```python
from build123d import *

# Parameters (mm, degrees)
SKETCH1_R           = 2.1
BOSS_EXTRUDE1_DEPTH = 500


with BuildPart() as part:
    # Sketch1 → Boss-Extrude1 (new body)
    with BuildSketch(Plane(origin=(0, 0, 0), x_dir=(-1, 0, 0), z_dir=(0, 0, -1))):
        with BuildLine():
            Line((-9.646446609, -22.821446609), (-7.771446609, -20.946446609))
            ThreePointArc((-7.771446609, -20.946446609), (-7.663060234, -20.784234935), (-7.625, -20.592893219))
            Line((-7.625, -20.592893219), (-7.625, -20.5))
            ThreePointArc((-7.625, -20.5), (-7.478553391, -20.146446609), (-7.125, -20))
            Line((-7.125, -20), (-3.3, -20))
            ThreePointArc((-3.3, -20), (-3.087867966, -19.912132034), (-3, -19.7))
            Line((-3, -19.7), (-3, -18))
            Line((-3, -18), (-6, -18))
            Line((-6, -18), (-6, -17.060660172))
            Line((-6, -17.060660172), (-2.939339828, -14))
            Line((-2.939339828, -14), (-0.3, -14))
            Line((-0.3, -14), (0, -13.7))
            Line((0, -13.7), (0.3, -14))
            Line((0.3, -14), (2.939339828, -14))
            Line((2.939339828, -14), (6, -17.060660172))
            Line((6, -17.060660172), (6, -18))
            Line((6, -18), (3, -18))
            Line((3, -18), (3, -19.7))
            ThreePointArc((3, -19.7), (3.087867966, -19.912132034), (3.3, -20))
            Line((3.3, -20), (9, -20))
            ThreePointArc((9, -20), (9.707106781, -19.707106781), (10, -19))
            Line((10, -19), (10, -13.3))
            ThreePointArc((10, -13.3), (9.912132034, -13.087867966), (9.7, -13))
            Line((9.7, -13), (8, -13))
            Line((8, -13), (8, -16))
            Line((8, -16), (7.060660172, -16))
            Line((7.060660172, -16), (4, -12.939339828))
            Line((4, -12.939339828), (4, -10.3))
            Line((4, -10.3), (3.7, -10))
            Line((3.7, -10), (4, -9.7))
            Line((4, -9.7), (4, -7.060660172))
            Line((4, -7.060660172), (7.060660172, -4))
            Line((7.060660172, -4), (8, -4))
            Line((8, -4), (8, -7))
            Line((8, -7), (9.7, -7))
            ThreePointArc((9.7, -7), (9.912132034, -6.912132034), (10, -6.7))
            Line((10, -6.7), (10, 6.7))
            ThreePointArc((10, 6.7), (9.912132034, 6.912132034), (9.7, 7))
            Line((9.7, 7), (8, 7))
            Line((8, 7), (8, 4))
            Line((8, 4), (7.060660172, 4))
            Line((7.060660172, 4), (4, 7.060660172))
            Line((4, 7.060660172), (4, 9.7))
            Line((4, 9.7), (3.7, 10))
            Line((3.7, 10), (4, 10.3))
            Line((4, 10.3), (4, 12.939339828))
            Line((4, 12.939339828), (7.060660172, 16))
            Line((7.060660172, 16), (8, 16))
            Line((8, 16), (8, 13))
            Line((8, 13), (9.7, 13))
            ThreePointArc((9.7, 13), (9.912132034, 13.087867966), (10, 13.3))
            Line((10, 13.3), (10, 19))
            ThreePointArc((10, 19), (9.707106781, 19.707106781), (9, 20))
            Line((9, 20), (3.300000001, 20))
            ThreePointArc((3.300000001, 20), (3.087867966, 19.912132034), (3, 19.699999999))
            Line((3, 19.699999999), (3, 18))
            Line((3, 18), (6, 18))
            Line((6, 18), (6, 17.060660172))
            Line((6, 17.060660172), (2.939339828, 14))
            Line((2.939339828, 14), (0.3, 14))
            Line((0.3, 14), (0, 13.7))
            Line((0, 13.7), (-0.3, 14))
            Line((-0.3, 14), (-2.939339828, 14))
            Line((-2.939339828, 14), (-6, 17.060660172))
            Line((-6, 17.060660172), (-6, 18))
            Line((-6, 18), (-3, 18))
            Line((-3, 18), (-3, 19.7))
            ThreePointArc((-3, 19.7), (-3.087867966, 19.912132034), (-3.3, 20))
            Line((-3.3, 20), (-7.125, 20))
            ThreePointArc((-7.125, 20), (-7.478553391, 20.146446609), (-7.625, 20.5))
            Line((-7.625, 20.5), (-7.625, 20.592893219))
            ThreePointArc((-7.625, 20.592893219), (-7.663060234, 20.784234935), (-7.771446609, 20.946446609))
            Line((-7.771446609, 20.946446609), (-9.646446609, 22.821446609))
            ThreePointArc((-9.646446609, 22.821446609), (-10, 22.967893219), (-10.353553391, 22.821446609))
            Line((-10.353553391, 22.821446609), (-12.228553391, 20.946446609))
            ThreePointArc((-12.228553391, 20.946446609), (-12.336939766, 20.784234935), (-12.375, 20.592893219))
            Line((-12.375, 20.592893219), (-12.375, 20))
            Line((-12.375, 20), (-10, 20))
            Line((-10, 20), (-10, 13.3))
            ThreePointArc((-10, 13.3), (-9.912132034, 13.087867966), (-9.7, 13))
            Line((-9.7, 13), (-8, 13))
            Line((-8, 13), (-8, 16))
            Line((-8, 16), (-7.060660172, 16))
            Line((-7.060660172, 16), (-4, 12.939339828))
            Line((-4, 12.939339828), (-4, 10.3))
            Line((-4, 10.3), (-3.7, 10))
            Line((-3.7, 10), (-4, 9.7))
            Line((-4, 9.7), (-4, 7.060660172))
            Line((-4, 7.060660172), (-7.060660172, 4))
            Line((-7.060660172, 4), (-8, 4))
            Line((-8, 4), (-8, 7))
            Line((-8, 7), (-9.7, 7))
            ThreePointArc((-9.7, 7), (-9.912132034, 6.912132034), (-10, 6.7))
            Line((-10, 6.7), (-10, -9.7))
            Line((-10, -9.7), (-9.7, -10))
            Line((-9.7, -10), (-10, -10.3))
            Line((-10, -10.3), (-10, -20))
            Line((-10, -20), (-12.375, -20))
            Line((-12.375, -20), (-12.375, -20.592893219))
            ThreePointArc((-12.375, -20.592893219), (-12.336939766, -20.784234935), (-12.228553391, -20.946446609))
            Line((-12.228553391, -20.946446609), (-10.353553391, -22.821446609))
            ThreePointArc((-10.353553391, -22.821446609), (-10, -22.967893219), (-9.646446609, -22.821446609))
        make_face()
        with Locations(Location((0, 10, 0), (0, 0, 180))):
            Circle(SKETCH1_R, mode=Mode.SUBTRACT)
        with Locations(Location((0, -10, 0), (0, 0, 180))):
            Circle(SKETCH1_R, mode=Mode.SUBTRACT)
        Polygon((-8, -4), (-7.060660172, -4), (-4, -7.060660172), (-4, -12.939339828), (-7.060660172, -16), (-8, -16), align=None, mode=Mode.SUBTRACT)
        Polygon((8, -2.5), (6.439339828, -2.5), (2.939339828, -6), (-2.939339828, -6), (-6.439339828, -2.5), (-8, -2.5), (-8, 2.5), (-6.439339828, 2.5), (-2.939339828, 6), (2.939339828, 6), (6.439339828, 2.5), (8, 2.5), align=None, mode=Mode.SUBTRACT)
    extrude(amount=-BOSS_EXTRUDE1_DEPTH)


solid = part.part
```
Can you work these out from the model? Positions are in its coordinate system, mm. A direction names the side the tool comes from. Coordinates: 2 decimals unless noted, no trailing zeros. Answer as CSV lines item,"result". Start each with the question number.
1) Thinking about a two-plate mould opening in Y: for faces 1 (the flat face through (10, -15, 246)), 2 (the flat face through (-10, 0, 246)), which applies, pulls with the +Y half, pulls with the -Y half, needs draft (parallel to the pull), parting line crosses it, or undercut?
2) For pin 1 (8 mm diameter, centred on y = 1, z = 270, fed in from +X); pin 2 (5 mm diameter, centred on x = 2.5, y = 1, fed in from +Z) (1 decimal); pin 3 (2 mm diameter, centred on x = -6.5, z = 70, fed in from +Y); pin 4 (0.8 mm diameter, centred on x = -1.5, z = 338, fed in from -Y), each with a flat end and sliding along its axis, tell me the tip position at first contact or that it passes through.
3) I need wall thicknesses on line 1 (X direction, y = -10, z = 140.5); line 2 (Y direction, x = 0, z = 291.5); line 3 (Y direction, x = 0.5, z = 457). Which ranges of each line are inside material? Lowest first, please. Write a range as from..to.
4) Suppose I cut it at A-A (z = 74). Count the separate pieces of the cut face and the enclosed holes in it, plus the area to 3 significant figures.
5) Which directions (+Z, -Z, +X, -X, +Y, -Y) give clear straight access to the entire face, cutting with the end or side of a thin tool? Please do faces 3 (the flat face through (10, -1, 246)), 4 (the flat face through (8, -10, 246)), 5 (the flat face through (5, -5, 500)).
Check result:
1,face 1,"undercut"
1,face 2,"needs draft"
2,pin 1,"stops at x = 10"
2,pin 2,"passes through"
2,pin 3,"stops at y = 20"
2,pin 4,"stops at y = -14"
3,line 1,"x = -3.7..-2.1, 2.1..4, 8..9.7"
3,line 2,"y = -13.7..-12.1, -7.9..-6, 6..7.9, 12.1..13.7"
3,line 3,"y = -14..-12.04, -7.96..-6, 6..7.96, 12.04..14"
4,separate pieces,"1"
4,enclosed holes,"4"
4,area,"353 mm²"
5,face 3,"+Z, -Z, +X"
5,face 4,"+Z, -Z"
5,face 5,"+Z, +X, -X, +Y, -Y"
